Autodesk Fusion 360 part; units mm, degrees
sketch "Schizzo5" plane through (0, 0, 0) normal (0, 0, 1) x (1, 0, 0)
  line L0 (84.2066, 82.4519) -> (84.2066, -13.5481)
  circle A0 centre (89.2066, -11.0481) radius 1.5
  circle A1 centre (129.2066, 79.9519) radius 3
  line L1 (84.2066, 34.4519) -> (134.2066, 34.4519) construction
  circle A2 centre (109.2066, 79.9519) radius 1.5
  circle A3 centre (89.2066, 79.9519) radius 3
  circle A4 centre (89.2066, 79.9519) radius 1.5
  line L2 (134.2066, 82.4519) -> (84.2066, 82.4519)
  circle A5 centre (129.2066, 79.9519) radius 1.5
  circle A6 centre (109.2066, 79.9519) radius 3
  circle A7 centre (109.2066, 34.4519) radius 4.1
  circle A8 centre (109.2066, -11.0481) radius 1.5
  line L3 (134.2066, -13.5481) -> (134.2066, 82.4519)
  line L4 (89.2066, 82.4519) -> (89.2066, -13.5481) construction
  circle A9 centre (89.2066, -11.0481) radius 3
  circle A10 centre (109.2066, -11.0481) radius 3
  circle A11 centre (129.2066, -11.0481) radius 1.5
  line L5 (84.2066, -13.5481) -> (134.2066, -13.5481)
  circle A12 centre (129.2066, -11.0481) radius 3
  line L6 (84.2066, -11.0481) -> (134.2066, -11.0481) construction
  line L7 (109.2066, 82.4519) -> (109.2066, -13.5481) construction
  line L8 (109.2066, 34.4519) -> (109.2066, 59.4519) construction
  line L9 (109.2066, 34.4519) -> (109.2066, 59.4519) construction
  line L10 (109.2066, 34.4519) -> (92.9431, 18.1884) construction
  circle A13 centre (92.9431, 18.1884) radius 4.1
  circle A14 centre (92.9431, 50.7153) radius 4.1
  circle A15 centre (125.47, 50.7153) radius 4.1
  circle A16 centre (125.47, 18.1884) radius 4.1
  circle A17 centre (109.2066, 34.4519) radius 18.9
  circle A18 centre (109.2066, 34.4519) radius 27.1
  point P0 (127.8474, 12.2366)
  dimension "d221" = 50
  dimension "d222" = 96
  dimension "d223" = 2.5
  dimension "d224" = 20
  dimension "d225" = 3
  dimension "d226" = 6
  dimension "d227" = 3
  dimension "d228" = 6
  dimension "d229" = 8.2
  dimension "d350" = 8.2
  dimension "d351" = 45
  dimension "d352" = 23
extrude "Estrusione24" add sketch "Schizzo5" along normal blind 5 contours L0 A1 A3 L2 A6 L3 A18 | L0 A13 A14 A17 A18 | L0 L3 A9 A10 L5 A12 A18 | A17 | L3 A15 A16 A17 A18
extrude "Estrusione25" add sketch "Schizzo5" along normal blind 1.8 contours A3 L2 | L2 A6 | A9 L5 | A1 L2 | A10 L5 | L5 A12 picked at (89.244, 82.1172) picked at (109.244, 82.1172) picked at (89.244, -13.2134) picked at (129.244, 82.1172) picked at (109.244, -13.2134) picked at (129.244, -13.2134)
equation "d225 = d227"
equation "d226 = d228"
equation "d350 = d229"
Geometry: final body of the model. Coordinates: model frame, mm. A direction names the side the tool comes from. Round coordinates to 2 decimals unless told otherwise and drop trailing zeros. Order: outer loops, then holes, each group sorted by start corner. A loop starts at its lowest first (then second) coordinate and runs counter-clockwise, first axis right, second up. Notation, with made-up numbers: (7.25, -5) -> (31.25, -5) arc R20 cw to (31.25, 11) -> close; hole circle Ø3 at (-8.5, 78.25). An arc over 180 degrees is marked (long way). Use one line per item in the form item = value.
(1) Access query for faces 4 (the face through (109, 53.35, 2.46)), 5 (the face through (84.207, 35, 2)), 6 (the face through (129.1, -8.05, 3.38)). Directions: +Z, -Z, +X, -X, +Y, -Y. A direction counts if a zero-diameter tool reaches every point of the face in a straight line with its end or side. Return the directions, or none.
Results list:
face_4 = +Z, -Z
face_5 = +Z, -Z, -X, +Y, -Y
face_6 = +Z
(2) Section A-A on x = 118. Return loops of the section in (y, z), and give its area (3 significant figures).
Results list:
outline = (-13.55, 0) -> (8.82, 0) -> (8.82, 5) -> (-13.55, 5) -> close; (17.72, 0) -> (51.18, 0) -> (51.18, 5) -> (17.72, 5) -> close; (60.09, 0) -> (82.45, 0) -> (82.45, 5) -> (60.09, 5) -> close
area = 391 mm^2
(3) Ray query, probe 1 along Y at (x, z) = (125.5, 1.7); probe 2 along Y at (x, z) = (90, 3.6); probe 3 along Y at (x, z) = (110.5, 1.35). Return the intervals inside material, ascending. Write a range as [from, to].
Results list:
probe_1 = [-13.55, 12.8], [22.29, 46.62], [56.11, 82.45]
probe_2 = [-8.15, 15.33], [21.04, 47.86], [53.57, 77.06]
probe_3 = [-13.55, -11.81], [-10.29, 7.38], [15.6, 30.56], [38.34, 53.31], [61.52, 79.19], [80.71, 82.45]
(4) Section D-D on y = 8.5. Return loops of the section in (x, z), and give its area (3 significant figures).
Results list:
outline = (84.21, 0) -> (101.4, 0) -> (101.4, 5) -> (84.21, 5) -> close; (117.01, 0) -> (134.21, 0) -> (134.21, 5) -> (117.01, 5) -> close
area = 172 mm^2
(5) Section C-C on z = 0.8. Count the separate pieces of the cut face and the enclosed holes in it, and give its area (3 significant figures).
Results list:
separate_pieces = 1
enclosed_holes = 9
area = 4,010 mm^2
(6) Section B-B on y = 59. Return loops of the section in (x, z).
Results list:
outline = (84.21, 0) -> (97.73, 0) -> (97.73, 5) -> (84.21, 5) -> close; (120.69, 0) -> (134.21, 0) -> (134.21, 5) -> (120.69, 5) -> close
(7) First-contact query: pin 1 Ø4.5 at (x, y) = (89, -11) entering from +Z; pin 2 Ø2.5 at (x, y) = (109.21, -11.05) entering from +Z. Flat tips, straight axial feed; report the tip coordinate or a pass-through.
Results list:
pin_1 = 1.8
pin_2 = through
(8) Draft query along Y for faces 1 (the face through (128.43, 47.88, 2.46)), 2 (the face through (103, 35, 5)), 3 (the face through (109, -13.548, 1)). Return one class per face: pulls with the +Y half, pulls with the -Y half, needs draft (parallel to the pull), parting line crosses it, or undercut.
Results list:
face_1 = undercut
face_2 = needs draft
face_3 = pulls with the -Y half
